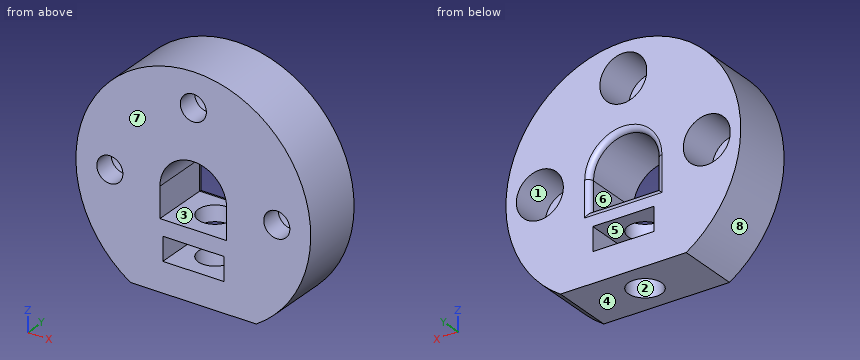
```python
from build123d import *

# Parameters (mm, degrees)
BOSS_EXTRU_1_DEPTH             = 6
CBORE_FOR_M2_SHCS1_D           = 2.5
CBORE_FOR_M2_SHCS1_CBORE_D     = 4.5
CBORE_FOR_M2_SHCS1_CBORE_DEPTH = 4
CONG_1_R                       = 0.5
ESQUISSE6_R                    = 1.6
ENL_V_MAT_EXTRU_1_DEPTH        = 18.003676108
ESQUISSE7_W                    = 5.85
ESQUISSE7_H                    = 2.25
ENL_V_MAT_EXTRU_2_DEPTH        = 7.25


with BuildPart() as part:
    # Esquisse1 → Boss.-Extru.1 (new body)
    with BuildSketch(Plane(origin=(0, 0, 0), x_dir=(1, 0, 0), z_dir=(0, 1, 0))):
        with BuildLine():
            Line((6.025985397, 9.5), (-6.025985397, 9.5))
            ThreePointArc((-6.025985397, 9.5), (0, -11.25), (6.025985397, 9.5))
        make_face()
        with BuildLine():
            Line((-3.2, 0), (-3.2, 2.9))
            Line((-3.2, 2.9), (3.2, 2.9))
            Line((3.2, 2.9), (3.2, 0))
            ThreePointArc((3.2, 0), (0, -3.2), (-3.2, 0))
        make_face(mode=Mode.SUBTRACT)
    extrude(amount=BOSS_EXTRU_1_DEPTH)

    # CBORE for M2 SHCS1 (through all)
    with Locations(Plane(origin=(0, 6, 0), x_dir=(1, 0, 0), z_dir=(0, 1, 0))):
        with Locations((8, 0), (-8, 0), (0, 0), (0, -8)):
            CounterBoreHole(CBORE_FOR_M2_SHCS1_D / 2, CBORE_FOR_M2_SHCS1_CBORE_D / 2, CBORE_FOR_M2_SHCS1_CBORE_DEPTH)

    # Congé1
    cong_1_edges = [part.edges().sort_by_distance(p)[0] for p in [
        (0, 6, 3.2),
        (3.2, 6, -1.45),
        (0, 6, -2.9),
        (-3.2, 6, -1.45),
    ]]
    fillet(cong_1_edges, radius=CONG_1_R)

    # Esquisse6 → Enlèv. mat.-Extru.1 (cut, through all)
    with BuildSketch(Plane.XY):
        with Locations((0, 3)):
            Circle(ESQUISSE6_R)
    extrude(amount=-ENL_V_MAT_EXTRU_1_DEPTH, mode=Mode.SUBTRACT)

    # Esquisse7 → Enlèv. mat.-Extru.2 (cut)
    with BuildSketch(Plane(origin=(0, 0, 0), x_dir=(1, 0, 0), z_dir=(0, 1, 0))):
        with Locations((0, 5.525)):
            Rectangle(ESQUISSE7_W, ESQUISSE7_H)
    extrude(amount=ENL_V_MAT_EXTRU_2_DEPTH, mode=Mode.SUBTRACT)


solid = part.part
```
Work out the finished part from the listing and answer in its coordinate system (mm). Face numbers are marked on the shaded views. A direction names the side the tool comes from. Round coordinates to 2 decimals unless told otherwise and drop trailing zeros. Order: outer loops, then holes, each group sorted by start corner. A loop starts at its lowest first (then second) coordinate and runs counter-clockwise, first axis right, second up.
Q1. A cutting plane is placed at D-D, the plane z = 8. Determine the outline of the cut face in (x, y), then the cut area to 3 significant figures.
Solution:
outline: (-7.91, 0) - (-1.25, 0) - (-1.25, 2) - (-2.25, 2) - (-2.25, 6) - (-7.91, 6) - close; (1.25, 0) - (7.91, 0) - (7.91, 6) - (2.25, 6) - (2.25, 2) - (1.25, 2) - close
area: 71.9 mm2
Q2. Given pin 1 Ø4 at (x, z) = (-8, 0) entering from +Y; pin 2 Ø1.4 at (y, z) = (3, -2) entering from -X; pin 3 Ø2.5 at (x, y) = (0, 3) entering from -Z, each flat-ended and moving along its own axis, determine where each tip first touches the part or whether it passes through.
Solution:
pin 1: stops at y = 2
pin 2: stops at x = -11.17
pin 3: stops at z = 2.95
Q3. The mould has two halves that part along Z. Classify the marked faces 5, 6, 7 and 8: pulls with the +Z half, pulls with the -Z half, needs draft (parallel to the pull), parting line crosses it, or undercut.
Solution:
face 5: undercut
face 6: undercut
face 7: needs draft
face 8: parting line crosses it
Q4. A cutting plane is placed at A-A, the plane z = -5.75. Determine the outline of the cut face in (x, y) (3 decimals).
Solution:
outline: (-9.67, 0) - (-2.925, 0) - (-2.925, 6) - (-9.67, 6) - close; (2.925, 0) - (9.67, 0) - (9.67, 6) - (2.925, 6) - close
Q5. Find the intervals of material crossed by line 1 along Y through (x, z) = (0, -8.6); line 2 along Z through (x, y) = (1, 5.75); line 3 along Z through (x, y) = (-0.5, 1.25), in increasing order.
Solution:
line 1: y = 0 to 1.4, 4.6 to 6
line 2: z = -9.5 to -6.65, -4.4 to -2.97, 3.11 to 5.98, 10.02 to 11.21
line 3: z = -9.5 to -6.65, -4.4 to -2.9, 3.16 to 6.85, 9.15 to 11.24
Q6. A cutting plane is placed at B-B, the plane y = 2.25. Determine the outline of the cut face in (x, z) (3 decimals).
Solution:
outline: (-6.026, -9.5) - (-1.413, -9.5) - (-1.413, -6.65) - (-2.925, -6.65) - (-2.925, -4.4) - (-1.413, -4.4) - (-1.413, -2.9) - (-3.2, -2.9) - (-3.2, 0) arc R3.2 cw to (3.2, 0) - (3.2, -2.9) - (1.413, -2.9) - (1.413, -4.4) - (2.925, -4.4) - (2.925, -6.65) - (1.413, -6.65) - (1.413, -9.5) - (6.026, -9.5) arc R11.25 ccw (long way) to start; hole circle Ø4.5 at (-8, 0); hole circle Ø4.5 at (0, 8); hole circle Ø4.5 at (8, 0)
Q7. A tool of negligible diameter and unlimited length cuts with its end or side. For the marked faces 1, 2, 3 and 4, from which of +Z, -Z, +X, -X, +Y, -Y can it reach the whole face along a straight path? Write none if from no direction.
Solution:
face 1: +Y
face 2: -Z
face 3: +Y, -Y
face 4: -Z, +X, -X, +Y, -Y
Q8. A cutting plane is placed at C-C, the plane x = -8. Determine the outline of the cut face in (y, z).
Solution:
outline: (0, -7.91) - (6, -7.91) - (6, -2.25) - (2, -2.25) - (2, -1.25) - (0, -1.25) - close; (0, 1.25) - (2, 1.25) - (2, 2.25) - (6, 2.25) - (6, 7.91) - (0, 7.91) - close
